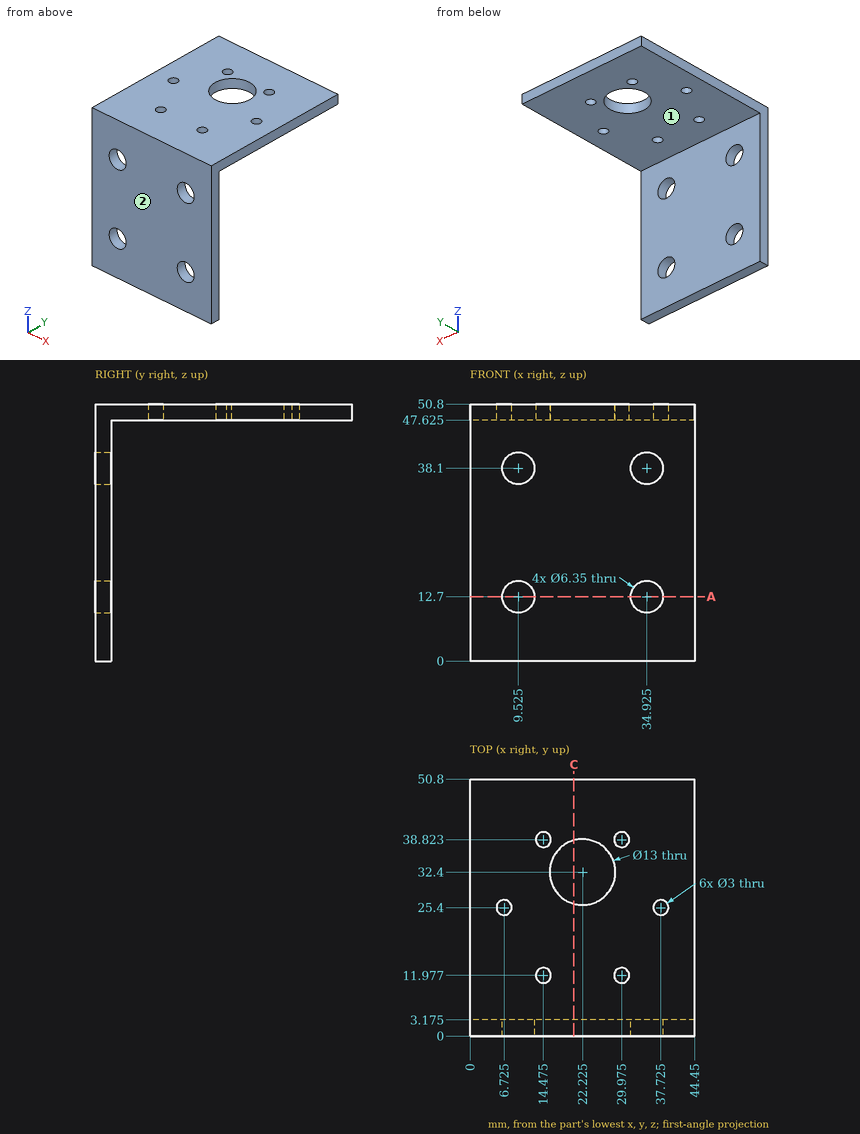
Verification items for this drawing (mm, ordinates from the low corner). A direction names the side the tool comes from. Coordinates: 2 decimals unless noted, no trailing zeros. Loops run counter-clockwise (first coordinate to the right, second up) from the corner with the lowest first, then second, coordinate; pieces in that order, holes last.
Item 1: Sectioned sample at A-A, the plane z = 12.7. Count the separate pieces of the cut face and the enclosed holes in it, then the cut area to 3 significant figures.
Item 2: Thickness scan on line 1 (Y direction, x = 24.5, z = 12.5) (1 decimal); line 2 (Z direction, x = 36, y = 25) (1 decimal). Record the ranges inside material, lowest first.
Item 3: Access from +Z, -Z, +X, -X, +Y, -Y to the whole of each face (thin tool, end or side, straight path). Record for the marked faces 1 and 2.
Item 4: Go/stop test with flat-tipped pins: pin 1 Ø17 at (x, y) = (22.225, 32.4) entering from -Z (3 decimals); pin 2 Ø8.5 at (x, z) = (9.525, 12.7) entering from +Y (3 decimals). Record where each tip stops, or that it passes through.
Item 5: Sectioned sample at C-C, the plane x = 20.5. Record the boundary of the cut face in (y, z) (1 decimal).
Check result:
1. separate pieces: 3
1. enclosed holes: 0
1. area: 101 mm2
2. line 1: y = 0 to 3.2
2. line 2: z = 47.6 to 50.8
3. face 1: -Z, +X, -X, +Y
3. face 2: +Z, -Z, +X, -X, -Y
4. pin 1: stops at z = 47.625
4. pin 2: stops at y = 3.175
5. outline: (0, 0) - (3.2, 0) - (3.2, 47.6) - (26.1, 47.6) - (26.1, 50.8) - (0, 50.8) - close; (38.7, 47.6) - (50.8, 47.6) - (50.8, 50.8) - (38.7, 50.8) - close
